Check sheet for the drawn part. Datum: minimum x, y, z corner. Units: mm. A direction names the side the tool comes from. Coordinates: 2 decimals unless noted, no trailing zeros. Order: outer loops, then holes, each group sorted by start corner. A loop starts at its lowest first (then second) coordinate and runs counter-clockwise, first axis right, second up. Notation, with made-up numbers: (-34, 37) - (-21, 37) arc R20 cw to (-21, 47) - close; hole circle Ø10 at (9, 68.25). An arc over 180 degrees is marked (long way). Answer as CSV lines item,"result". Start each with the question number.
1. Mould release check, pull along X, two halves, no side actions. Record for the marked faces 1, 2 and 3: pulls with the +X half, pulls with the -X half, needs draft (parallel to the pull), parting line crosses it, or undercut.
2. Section check C-C (z = 4). Record the cut outline in (x, y), and give its area (3 significant figures).
3. Section check A-A (y = 6.25). Record the cut outline in (x, z), and give its area (3 significant figures).
4. Section check B-B (z = 29). Record the cut outline in (x, y).
5. Section check D-D (x = 7). Record the cut outline in (y, z).
6. Set-up check for the marked faces 4 and 5: record each of +Z, -Z, +X, -X, +Y, -Y from which the full face is reachable in a straight line by a thin tool's end or side.
7. Go/stop test with flat-tipped pins: pin 1 (1.1 mm diameter, centred on x = 28, y = 15.5, fed in from +Z); pin 2 (2 mm diameter, centred on x = 24.5, y = 4, fed in from +Z); pin 3 (8 mm diameter, centred on x = 18, z = 19.5, fed in from -Y). Record where each tip stops, or that it passes through.
8. Material ranges on L1, parallel to Z at x = 8, y = 5.25; L2, parallel to X at y = 1.25, z = 28; L3, parallel to Y at x = 33.5, z = 6.5, recorded low to high. Write a range as [from, to].
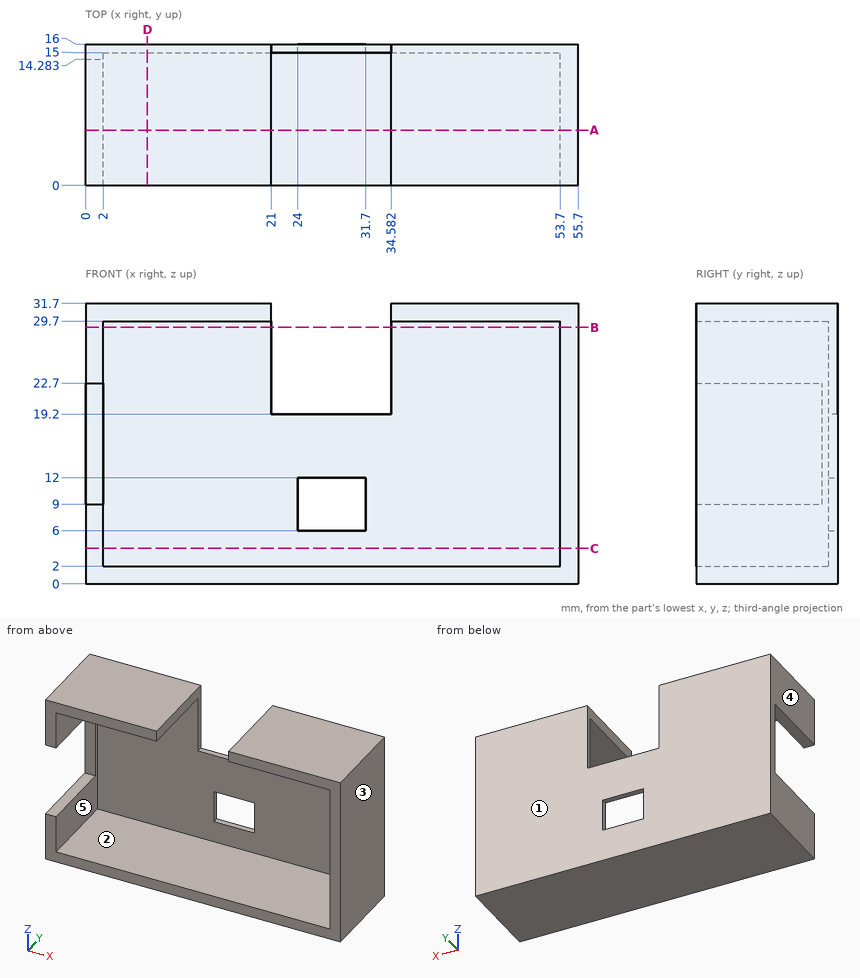
Evaluation:
1,face 1,"needs draft"
1,face 2,"undercut"
1,face 3,"pulls with the +X half"
2,outline,"(0, 0) - (2, 0) - (2, 15) - (53.7, 15) - (53.7, 0) - (55.7, 0) - (55.7, 16) - (0, 16) - close"
2,area,"116 mm²"
3,outline,"(0, 0) - (55.7, 0) - (55.7, 31.7) - (34.58, 31.7) - (34.58, 29.7) - (53.7, 29.7) - (53.7, 2) - (2, 2) - (2, 9) - (0, 9) - close; (0, 22.7) - (2, 22.7) - (2, 29.7) - (21, 29.7) - (21, 31.7) - (0, 31.7) - close"
3,area,"279 mm²"
4,outline,"(0, 0) - (2, 0) - (2, 15) - (21, 15) - (21, 16) - (0, 16) - close; (34.58, 15) - (53.7, 15) - (53.7, 0) - (55.7, 0) - (55.7, 16) - (34.58, 16) - close"
5,outline,"(0, 0) - (16, 0) - (16, 31.7) - (0, 31.7) - (0, 29.7) - (15, 29.7) - (15, 2) - (0, 2) - close"
6,face 4,"+Z, -Z, -X, +Y, -Y"
6,face 5,"-Y"
7,pin 1,"stops at z = 19.2"
7,pin 2,"stops at z = 2"
7,pin 3,"stops at y = 15"
8,L1,"z = [0, 2], [29.7, 31.7]"
8,L2,"x = [0, 2], [53.7, 55.7]"
8,L3,"y = [15, 16]"
